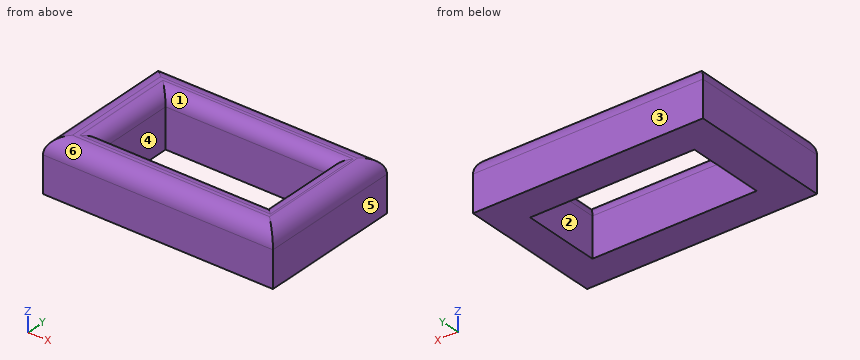
```python
from build123d import *

# Parameters (mm, degrees)
F0_W     = 35
F0_H     = 22
F0_W_2   = 25
F0_H_2   = 12
F1_DEPTH = 8
F2_R     = 2.5
F3_R     = 2


with BuildPart() as f1:
    # F0 (on Top) → F1 (new body)
    with BuildSketch(Plane.XY):
        with Locations((-41.790893, 40.325698)):
            Rectangle(F0_W, F0_H)
        with Locations((-41.567577, 40.353398)):
            Rectangle(F0_W_2, F0_H_2, mode=Mode.SUBTRACT)
    extrude(amount=F1_DEPTH)

    # F2
    f2_edges = [f1.edges().sort_by_distance(p)[0] for p in [
        (-41.790893, 29.325698, 8),
        (-59.290893, 40.325698, 8),
        (-41.790893, 51.325698, 8),
        (-24.290893, 40.325698, 8),
    ]]
    fillet(f2_edges, radius=F2_R)

    # F3
    f3_edges = [f1.edges().sort_by_distance(p)[0] for p in [
        (-41.567577, 46.353398, 8),
        (-54.067577, 40.353398, 8),
        (-41.567577, 34.353398, 8),
        (-29.067577, 40.353398, 8),
    ]]
    fillet(f3_edges, radius=F3_R)


solid = f1.part
```
Build history of the part. All positions in model axes, mm. Face numbers are marked on the shaded views. A direction names the side the tool comes from. Round coordinates to 2 decimals unless told otherwise and drop trailing zeros. Order: outer loops, then holes, each group sorted by start corner. A loop starts at its lowest first (then second) coordinate and runs counter-clockwise, first axis right, second up. Notation, with made-up numbers: (-12, 30.5) - (12, 30.5) arc R22 ccw to (12, 52.5) - close; hole circle Ø4 at (20, 11.5). An arc over 180 degrees is marked (long way). Use a Markdown table: item, result.
1) Saw through at B-B on x = -44. Write the cut outline in (y, z).
Recorded:
| item | result |
|---|---|
| outline | (29.33, 0) - (34.35, 0) - (34.35, 6) arc R2 ccw to (32.35, 8) - (31.83, 8) arc R2.5 ccw to (29.33, 5.5) - close; (46.35, 0) - (51.33, 0) - (51.33, 5.5) arc R2.5 ccw to (48.83, 8) - (48.35, 8) arc R2 ccw to (46.35, 6) - close |
2) Saw through at A-A on z = 4.5. Write the cut outline in (x, y).
Recorded:
| item | result |
|---|---|
| outline | (-59.29, 29.33) - (-24.29, 29.33) - (-24.29, 51.33) - (-59.29, 51.33) - close; hole (-54.07, 34.35) - (-29.07, 34.35) - (-29.07, 46.35) - (-54.07, 46.35) - close |
3) Wall check: L1, parallel to Y at x = -36, z = 4.5; L2, parallel to X at y = 44, z = 5.25; L3, parallel to Y at x = -43, z = 7. Give the ranges that are in metal, low to high.
Recorded:
| item | result |
|---|---|
| L1 | y = 29.33 to 34.35, 46.35 to 51.33 |
| L2 | x = -59.29 to -54.07, -29.07 to -24.29 |
| L3 | y = 29.83 to 34.09, 46.62 to 50.83 |
4) Saw through at C-C on y = 43.5. Write the cut outline in (x, z).
Recorded:
| item | result |
|---|---|
| outline | (-59.29, 0) - (-54.07, 0) - (-54.07, 6) arc R2 ccw to (-56.07, 8) - (-56.79, 8) arc R2.5 ccw to (-59.29, 5.5) - close; (-29.07, 0) - (-24.29, 0) - (-24.29, 5.5) arc R2.5 ccw to (-26.79, 8) - (-27.07, 8) arc R2 ccw to (-29.07, 6) - close |
5) Tool access for the marked faces 1, 2 and 3: list every direction of +Z, -Z, +X, -X, +Y, -Y with a clear straight run to the whole face (end or side of a thin tool).
Recorded:
| item | result |
|---|---|
| face 1 | +Z |
| face 2 | +Z, -Z |
| face 3 | +Z, -Z, +X, -X, +Y |
6) Saw through at D-D on z = 7.25. Write the cut outline in (x, y).
Recorded:
| item | result |
|---|---|
| outline | (-58.58, 30.04) - (-25.01, 30.04) - (-25.01, 50.61) - (-58.58, 50.61) - close; hole (-54.51, 33.91) - (-28.63, 33.91) - (-28.63, 46.79) - (-54.51, 46.79) - close |
7) Pull direction Y, two halves, no side cores. Call the marked faces 4, 5 and 6: pulls with the +Y half, pulls with the -Y half, needs draft (parallel to the pull), parting line crosses it, or undercut.
Recorded:
| item | result |
|---|---|
| face 4 | undercut |
| face 5 | needs draft |
| face 6 | pulls with the -Y half |
8) Flat gauge pins, fed straight in: pin 1 Ø1 at (y, z) = (41, 7) entering from +X; pin 2 Ø1.5 at (y, z) = (37.5, 6.5) entering from -X. Where does each tip first touch, or does it go through?
Recorded:
| item | result |
|---|---|
| pin 1 | stops at x = -24.5 |
| pin 2 | stops at x = -59.28 |
